```python
from build123d import *

# Parameters (mm, degrees)
F0_W     = 1.5233159065
F0_H     = 2
F0_W_2   = 2
F0_H_2   = 1.5
F0_W_3   = 1.4766840935
F1_DEPTH = 21.1
F2_R     = 3.0488114631
F3_DEPTH = 1
F4_R     = 2.4979644643
F5_DEPTH = 1.9
F6_R     = 0.2


with BuildPart() as f1:
    # F0 (on Top) → F1 (new body)
    with BuildSketch(Plane.XY):
        with Locations((-17.0561056584, 21.1294589788)):
            Rectangle(F0_W, F0_H)
        with Locations((-15.2944477051, 22.8794589788)):
            Rectangle(F0_W_2, F0_H_2)
        with Locations((-15.2944477051, 21.1294589788)):
            Rectangle(F0_W_2, F0_H)
        with Locations((-13.5561056584, 21.1294589788)):
            Rectangle(F0_W_3, F0_H)
        with Locations((-15.2944477051, 19.3794589788)):
            Rectangle(F0_W_2, F0_H_2)
    extrude(amount=F1_DEPTH)

    # F2 (on Top) → F3 (join)
    with BuildSketch(Plane.XY):
        with Locations((-15.3177636117, 21.1294589788)):
            Circle(F2_R)
    extrude(amount=-F3_DEPTH)

    # F4 (on face) → F5 (join)
    with BuildSketch(Plane(origin=(0, 0, -1), x_dir=(1, 0, 0), z_dir=(0, 0, -1))):
        with Locations((-15.3177636117, -21.1294589788)):
            Circle(F4_R)
    extrude(amount=F5_DEPTH)

    # F6
    f6_edges = [f1.edges().sort_by_distance(p)[0] for p in [
        (-12.817764, 20.129459, 10.55),
        (-12.817764, 22.129459, 10.55),
        (-14.294448, 18.629459, 10.55),
        (-16.294448, 18.629459, 10.55),
        (-17.817764, 20.129459, 10.55),
        (-17.817764, 22.129459, 10.55),
        (-16.294448, 23.629459, 10.55),
        (-14.294448, 23.629459, 10.55),
    ]]
    fillet(f6_edges, radius=F6_R)


solid = f1.part
```
Verification items for the finished model (mm, model axes). A direction names the side the tool comes from. Coordinates: 2 decimals unless noted, no trailing zeros. Loops run counter-clockwise (first coordinate to the right, second up) from the corner with the lowest first, then second, coordinate; pieces in that order, holes last. Notation, with made-up numbers: (-14, 11) - (17, 11) arc R21 cw to (17, 17) - close; hole circle Ø5 at (63, 59). An arc over 180 degrees is marked (long way). Put each result on its own line as item: value.
Item 1: Gauge pin test, flat ends, axial feed: pin 1 Ø1.3 at (y, z) = (21.5, 5.5) entering from +X; pin 2 Ø0.7 at (y, z) = (19.5, 8.5) entering from -X; pin 3 Ø1.8 at (x, z) = (-15, 12) entering from -Y. Record the tip position at first contact, or that the pin passes through.
Conclusion:
pin 1: stops at x = -12.82
pin 2: stops at x = -16.29
pin 3: stops at y = 18.63
Item 2: Section check B-B (x = -16.75). Enter the section's corners in (y, z).
Conclusion:
outline: (18.44, -1) - (19.08, -1) - (19.08, -2.9) - (23.18, -2.9) - (23.18, -1) - (23.82, -1) - (23.82, 0) - (22.13, 0) - (22.13, 21.1) - (20.13, 21.1) - (20.13, 0) - (18.44, 0) - close
Item 3: Section check A-A (z = 6.5). Enter the section's corners in (x, y), then the cut area to 3 significant figures.
Conclusion:
outline: (-17.82, 20.33) arc R0.2 ccw to (-17.62, 20.13) - (-16.29, 20.13) - (-16.29, 18.83) arc R0.2 ccw to (-16.09, 18.63) - (-14.49, 18.63) arc R0.2 ccw to (-14.29, 18.83) - (-14.29, 20.13) - (-13.02, 20.13) arc R0.2 ccw to (-12.82, 20.33) - (-12.82, 21.93) arc R0.2 ccw to (-13.02, 22.13) - (-14.29, 22.13) - (-14.29, 23.43) arc R0.2 ccw to (-14.49, 23.63) - (-16.09, 23.63) arc R0.2 ccw to (-16.29, 23.43) - (-16.29, 22.13) - (-17.62, 22.13) arc R0.2 ccw to (-17.82, 21.93) - close
area: 15.9 mm2
Item 4: Scan lines: line 1 along X through (y, z) = (20, 9); line 2 along Z through (x, y) = (-14, 23.5); line 3 along X through (y, z) = (20.5, 17.25). Record each from-to range of solid material in increasing order.
Conclusion:
line 1: x = -16.29 to -14.29
line 2: z = -1 to 0
line 3: x = -17.82 to -12.82
Item 5: Section check C-C (y = 21.5). Enter the section's corners in (x, z).
Conclusion:
outline: (-18.34, -1) - (-17.79, -1) - (-17.79, -2.9) - (-12.85, -2.9) - (-12.85, -1) - (-12.29, -1) - (-12.29, 0) - (-12.82, 0) - (-12.82, 21.1) - (-17.82, 21.1) - (-17.82, 0) - (-18.34, 0) - close
Item 6: Set-up check for faces 1 (the face through (-17, 22.129, 10)), 2 (the face through (-15, 23.629, 10)), 3 (the face through (-14.294, 19, 10)), 4 (the face through (-12.818, 21, 10)): record each of +Z, -Z, +X, -X, +Y, -Y from which the full face is reachable in a straight line by a thin tool's end or side.
Conclusion:
face 1: +Z, -X, +Y
face 2: +Z, +X, -X, +Y
face 3: +Z, +X, -Y
face 4: +Z, +X, +Y, -Y
